Autodesk Inventor part; units mm, degrees
ref_plane "YZ Plane" through (0, 0, 0) normal (1, 0, 0) x (0, 1, 0)
ref_plane "XZ Plane" through (0, 0, 0) normal (0, 1, 0) x (-1, 0, 0)
ref_plane "XY Plane" through (0, 0, 0) normal (0, 0, 1) x (1, 0, 0)
sketch "C3,5-8, 100uF_213" plane through (0, 0, 0) normal (0, 0, 1) x (1, 0, 0)
  line L0 (-3.994, 0.7945) -> (-3.8561, 1.309)
  line L1 (-3.8561, 1.309) -> (-3.6523, 1.8011)
  line L2 (-3.6523, 1.8011) -> (-3.3859, 2.2624)
  line L3 (-3.3859, 2.2624) -> (-3.0617, 2.685)
  line L4 (-3.0617, 2.685) -> (-2.685, 3.0617)
  line L5 (-2.685, 3.0617) -> (-2.2624, 3.3859)
  line L6 (-2.2624, 3.3859) -> (-1.8011, 3.6523)
  line L7 (-1.8011, 3.6523) -> (-1.309, 3.8561)
  line L8 (-1.309, 3.8561) -> (-0.7945, 3.994)
  line L9 (-0.7945, 3.994) -> (-0.2663, 4.0635)
  line L10 (-0.2663, 4.0635) -> (0, 4.0635)
  line L11 (0, 4.0635) -> (0.2663, 4.0635)
  line L12 (0.2663, 4.0635) -> (0.7944, 3.994)
  line L13 (0.7944, 3.994) -> (1.309, 3.8561)
  line L14 (1.309, 3.8561) -> (1.8011, 3.6523)
  line L15 (1.8011, 3.6523) -> (2.2624, 3.3859)
  line L16 (2.2624, 3.3859) -> (2.685, 3.0617)
  line L17 (2.685, 3.0617) -> (3.0616, 2.685)
  line L18 (3.0616, 2.685) -> (3.3859, 2.2624)
  line L19 (3.3859, 2.2624) -> (3.6522, 1.8011)
  line L20 (3.6522, 1.8011) -> (3.8561, 1.309)
  line L21 (3.8561, 1.309) -> (3.994, 0.7945)
  line L22 (3.994, 0.7945) -> (4.0635, 0.2663)
  line L23 (4.0635, 0.2663) -> (4.0635, -0.2663)
  line L24 (4.0635, -0.2663) -> (3.994, -0.7944)
  line L25 (3.994, -0.7944) -> (3.8561, -1.309)
  line L26 (3.8561, -1.309) -> (3.6522, -1.8011)
  line L27 (3.6522, -1.8011) -> (3.3859, -2.2624)
  line L28 (3.3859, -2.2624) -> (3.0616, -2.685)
  line L29 (3.0616, -2.685) -> (2.685, -3.0616)
  line L30 (2.685, -3.0616) -> (2.2624, -3.3859)
  line L31 (2.2624, -3.3859) -> (1.8011, -3.6522)
  line L32 (1.8011, -3.6522) -> (1.309, -3.8561)
  line L33 (1.309, -3.8561) -> (0.7944, -3.994)
  line L34 (0.7944, -3.994) -> (0.2663, -4.0635)
  line L35 (0.2663, -4.0635) -> (0, -4.0635)
  line L36 (0, -4.0635) -> (-0.2663, -4.0635)
  line L37 (-0.2663, -4.0635) -> (-0.7945, -3.994)
  line L38 (-0.7945, -3.994) -> (-1.309, -3.8561)
  line L39 (-1.309, -3.8561) -> (-1.8011, -3.6522)
  line L40 (-1.8011, -3.6522) -> (-2.2624, -3.3859)
  line L41 (-2.2624, -3.3859) -> (-2.685, -3.0616)
  line L42 (-2.685, -3.0616) -> (-3.0617, -2.685)
  line L43 (-3.0617, -2.685) -> (-3.3859, -2.2624)
  line L44 (-3.3859, -2.2624) -> (-3.6523, -1.8011)
  line L45 (-3.6523, -1.8011) -> (-3.8561, -1.309)
  line L46 (-3.8561, -1.309) -> (-3.994, -0.7944)
  line L47 (-3.994, -0.7944) -> (-4.0635, -0.2663)
  line L48 (-4.0635, -0.2663) -> (-4.0635, 0.2663)
  line L49 (-4.0635, 0.2663) -> (-3.994, 0.7945)
extrude "Extrusion1" add sketch "C3,5-8, 100uF_213" along normal blind 13
properties part number "100uF"
Input: part model. Units: mm. Frame: model coordinates. Give positions to 0.01 mm unless a question says otherwise; leave off trailing zeros. Loops run counter-clockwise (first coordinate to the right, second up) from the corner with the lowest first, then second, coordinate; pieces in that order, holes last. Notation, with made-up numbers: (76, 47) -> (107, 47) arc R18 ccw to (107, 79) -> close; hole circle Ø11 at (-18, 64). An arc over 180 degrees is marked (long way). Use a Markdown table: item, result.
Q1. First-contact query: P1, Ø2, axis at x = -2, y = -0.5, coming from the -Z side. Flat tip, straight axial feed; report the tip coordinate or a pass-through.
Entries:
| item | result |
|---|---|
| P1 | stops at z = 0 |
Q2. Ray query, probe 1 along Y at (x, z) = (1.25, 6.5); probe 2 along Y at (x, z) = (0.75, 10); probe 3 along X at (y, z) = (-1, 2.5). Return the intervals inside material, ascending. Write a range as from..to.
Entries:
| item | result |
|---|---|
| probe 1 | y = -3.87..3.87 |
| probe 2 | y = -4..4 |
| probe 3 | x = -3.94..3.94 |
Q3. Section query A-A, the plane y = -1.5. Return the cut outline in (x, z).
Entries:
| item | result |
|---|---|
| outline | (-3.78, 0) -> (3.78, 0) -> (3.78, 13) -> (-3.78, 13) -> close |
